Source: CAD feature listing. Evaluate the final solid. Frame: model axes, mm. A direction names the side the tool comes from. Round coordinates to 2 decimals unless told otherwise and drop trailing zeros. Order: outer loops, then holes, each group sorted by start corner. A loop starts at its lowest first (then second) coordinate and runs counter-clockwise, first axis right, second up.
```python
from build123d import *

# Parameters (mm, degrees)
BOSS_EXTRUDE1_DEPTH = 55
BOSS_EXTRUDE2_START = 2
BOSS_EXTRUDE2_DEPTH = 2
BOSS_EXTRUDE3_START = 2
BOSS_EXTRUDE3_DEPTH = 2
BOSS_EXTRUDE5_START = 2
BOSS_EXTRUDE5_DEPTH = 2
BOSS_EXTRUDE6_DEPTH = 2
SKETCH7_W           = 3.4
SKETCH7_H           = 11.3
CUT_EXTRUDE2_DEPTH  = 55


with BuildPart() as part:
    # Sketch1 → Boss-Extrude1 (new body)
    with BuildSketch(Plane.XY):
        with BuildLine():
            Line((0, 0), (0, -89.2))
            Line((0, -89.2), (-6, -89.2))
            Line((-6, -89.2), (-6, -79.2))
            Line((-6, -79.2), (-16, -79.2))
            Line((-16, -79.2), (-16, -72.2))
            ThreePointArc((-16, -72.2), (-8.4, -64.6), (-16, -57))
            Line((-16, -57), (-16, -42.3))
            Line((-16, -42.3), (-8.4, -42.3))
            Line((-8.4, -42.3), (-8.4, -35.6))
            Line((-8.4, -35.6), (-16, -35.6))
            Line((-16, -35.6), (-16, -32.2))
            ThreePointArc((-16, -32.2), (-8.4, -24.6), (-16, -17))
            Line((-16, -17), (-16, -10))
            Line((-16, -10), (-6, -10))
            Line((-6, -10), (-6, 0))
            Line((-6, 0), (0, 0))
        make_face()
    extrude(amount=BOSS_EXTRUDE1_DEPTH)

    # Sketch2 → Boss-Extrude2 (add)
    with BuildSketch(Plane(origin=(0, 0, 28.5), x_dir=(-1, 0, 0), z_dir=(0, 0, -1)).offset(BOSS_EXTRUDE2_START)):
        with BuildLine():
            Line((16, -32.2), (16, -29.5))
            ThreePointArc((16, -29.5), (11.1, -24.6), (16, -19.7))
            Line((16, -19.7), (16, -17))
            ThreePointArc((16, -17), (8.4, -24.6), (16, -32.2))
        make_face()
    extrude(amount=-BOSS_EXTRUDE2_DEPTH)

    # Sketch3 → Boss-Extrude3 (add)
    with BuildSketch(Plane(origin=(0, 0, 28.5), x_dir=(-1, 0, 0), z_dir=(0, 0, -1)).offset(BOSS_EXTRUDE3_START)):
        with BuildLine():
            Line((16, -72.2), (16, -69.5))
            ThreePointArc((16, -69.5), (11.1, -64.6), (16, -59.7))
            Line((16, -59.7), (16, -57))
            ThreePointArc((16, -57), (8.4, -64.6), (16, -72.2))
        make_face()
    extrude(amount=-BOSS_EXTRUDE3_DEPTH)

    # Sketch4 → Boss-Extrude5 (add)
    with BuildSketch(Plane(origin=(0, 0, 2), x_dir=(-1, 0, 0), z_dir=(0, 0, -1)).offset(BOSS_EXTRUDE5_START)):
        with BuildLine():
            Line((16, -57), (16, -59.7))
            ThreePointArc((16, -59.7), (11.1, -64.6), (16, -69.5))
            Line((16, -69.5), (16, -72.2))
            ThreePointArc((16, -72.2), (8.4, -64.6), (16, -57))
        make_face()
        with BuildLine():
            Line((16, -17), (16, -19.7))
            ThreePointArc((16, -19.7), (11.1, -24.6), (16, -29.5))
            Line((16, -29.5), (16, -32.2))
            ThreePointArc((16, -32.2), (8.4, -24.6), (16, -17))
        make_face()
    extrude(amount=-BOSS_EXTRUDE5_DEPTH)

    # Sketch5 → Boss-Extrude6 (add)
    with BuildSketch(Plane(origin=(0, 0, 53), x_dir=(-1, 0, 0), z_dir=(0, 0, -1))):
        with BuildLine():
            Line((16, -17), (16, -19.7))
            ThreePointArc((16, -19.7), (11.1, -24.6), (16, -29.5))
            Line((16, -29.5), (16, -32.2))
            ThreePointArc((16, -32.2), (8.4, -24.6), (16, -17))
        make_face()
        with BuildLine():
            Line((16, -57), (16, -59.7))
            ThreePointArc((16, -59.7), (11.1, -64.6), (16, -69.5))
            Line((16, -69.5), (16, -72.2))
            ThreePointArc((16, -72.2), (8.4, -64.6), (16, -57))
        make_face()
    extrude(amount=-BOSS_EXTRUDE6_DEPTH)

    # Sketch7 → Cut-Extrude2 (cut)
    with BuildSketch(Plane.XY.offset(55)):
        with Locations((-14.3, -47.95)):
            Rectangle(SKETCH7_W, SKETCH7_H)
    extrude(amount=-CUT_EXTRUDE2_DEPTH, mode=Mode.SUBTRACT)


solid = part.part
```
1. Section C-C on x = -13.5. State how many separate pieces and enclosed holes the cut face has, plus the area to 3 significant figures.
2. Access query for faces 1 (the face through (-16, -34, 27)), 2 (the face through (-12, -35.6, 27)), 3 (the face through (-10, -64, 26.5)). Directions: +Z, -Z, +X, -X, +Y, -Y. A direction counts if a zero-diameter tool reaches every point of the face in a straight line with its end or side. Return the directions, or none.
3. Pull-direction query (Z, two-part tool) for faces 4 (the face through (-11.1, -24.7, 27.5)), 5 (the face through (-10, -64, 28.5)), 6 (the face through (-6, -44, 55)); classes: released by +Z, released by -Z, zero draft, split by the parting line, or undercut.
4. Section A-A on z = 36. Return loops of the section in (x, y).
5. First-contact query: pin 1 (4 mm diameter, centred on x = -10, z = 38.5, fed in from -Y); pin 2 (1.3 mm diameter, centred on x = -11, z = 18, fed in from +Y); pin 3 (5.5 mm diameter, centred on y = -49, z = 14.5, fed in from -X); pin 4 (1.5 mm diameter, centred on x = -14, y = -25.5, fed in from +Z). Flat tips, straight axial feed; report the tip coordinate or a pass-through.
6. Line query: line 1 along Z through (x, y) = (-11.75, -62); line 2 along Y through (x, z) = (-11, 3); line 3 along X through (y, z) = (-6, 18). Output: solid intervals per line, ascending.
7. Section B-B on y = -24.6. Return loops of the section in (x, z), plus the area to 3 significant figures.
8. Section D-D on y = -38. Return loops of the section in (x, z).
Result:
1. separate pieces: 4
1. enclosed holes: 0
1. area: 1,310 mm2
2. face 1: +Z, -Z, -X, +Y, -Y
2. face 2: +Z, -Z, -X
2. face 3: -X
3. face 4: zero draft
3. face 5: undercut
3. face 6: released by +Z
4. outline: (-16, -79.2) - (-6, -79.2) - (-6, -89.2) - (0, -89.2) - (0, 0) - (-6, 0) - (-6, -10) - (-16, -10) - (-16, -17) arc R7.6 cw to (-16, -32.2) - (-16, -35.6) - (-8.4, -35.6) - (-8.4, -42.3) - (-12.6, -42.3) - (-12.6, -53.6) - (-16, -53.6) - (-16, -57) arc R7.6 cw to (-16, -72.2) - close
5. pin 1: stops at y = -79.2
5. pin 2: stops at y = -10
5. pin 3: stops at x = -12.6
5. pin 4: passes through
6. line 1: z = 0 to 2, 26.5 to 28.5, 53 to 55
6. line 2: y = -79.2 to -70.32, -58.88 to -42.3, -35.6 to -30.32, -18.88 to -10
6. line 3: x = -6 to 0
7. outline: (-11.1, 0) - (0, 0) - (0, 55) - (-11.1, 55) - (-11.1, 53) - (-8.4, 53) - (-8.4, 28.5) - (-11.1, 28.5) - (-11.1, 26.5) - (-8.4, 26.5) - (-8.4, 2) - (-11.1, 2) - close
7. area: 478 mm2
8. outline: (-8.4, 0) - (0, 0) - (0, 55) - (-8.4, 55) - close
